from build123d import *

# Parameters (mm, degrees)
F1_DEPTH = 28.575


# Not quite as in the source:
# - a feature names something its author has since deleted; it is built from what else it names


with BuildPart() as f1:
    # F0 (on Top) → F1 (new body)
    with BuildSketch(Plane.XY):
        with BuildLine():
            Line((1102.0184274855, 685.8), (-1143, 685.8))
            Line((-1143, 685.8), (-1143, 0))
            Line((-1143, 0), (88.9, 0))
            Line((88.9, 0), (88.9, 124.587))
            Line((88.9, 124.587), (292.1, 124.587))
            Line((292.1, 124.587), (292.1, 0))
            Line((292.1, 0), (1143, 0))
            Line((1143, 0), (1295.4, 0))
            ThreePointArc((1295.4, 0), (1261.244047213, 330.8283905438), (1160.2171388114, 647.7))
            ThreePointArc((1160.2171388114, 647.7), (1136.7988098871, 675.4279116849), (1102.0184274855, 685.8))
        make_face()
        with BuildLine():
            Line((88.9, 0), (-1143, 0))
            Line((-1143, 0), (-1143, -685.8))
            Line((-1143, -685.8), (1102.0184274855, -685.8))
            ThreePointArc((1102.0184274855, -685.8), (1136.7988098871, -675.4279116849), (1160.2171388114, -647.7))
            ThreePointArc((1160.2171388114, -647.7), (1261.244047213, -330.8283905438), (1295.4, 0))
            Line((1295.4, 0), (1143, 0))
            Line((1143, 0), (292.1, 0))
            Line((292.1, 0), (292.1, -124.587))
            Line((292.1, -124.587), (88.9, -124.587))
            Line((88.9, -124.587), (88.9, 0))
        make_face()
    extrude(amount=F1_DEPTH)


solid = f1.part
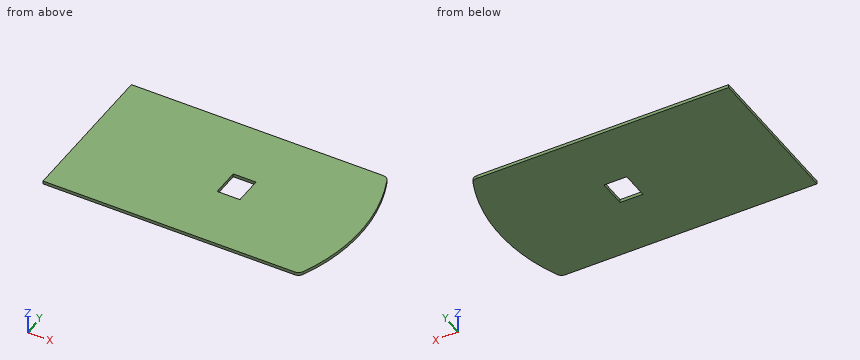
Can you work these out from the model? Positions are in its coordinate system, mm. Give positions to 0.01 mm unless a question says otherwise; leave off trailing zeros. Loops run counter-clockwise (first coordinate to the right, second up) from the corner with the lowest first, then second, coordinate; pieces in that order, holes last. Notation, with made-up numbers: M 70.25,17 L 112.25,17 A36 ccw 112.25,54 Z; hole C -23,10.5 d8. An arc over 180 degrees is marked long. One line per item, written item: value.
1) Imagine slicing it at A-A on z = 10. Write out the boundary of the cut face in (x, y).
Geometry check:
outline: M -1143,-685.8 L 1102.02,-685.8 A63.5 ccw 1160.22,-647.7 A1619.25 ccw 1160.22,647.7 A63.5 ccw 1102.02,685.8 L -1143,685.8 Z; hole M 88.9,-124.59 L 292.1,-124.59 L 292.1,124.59 L 88.9,124.59 Z
2) Imagine slicing it at D-D on y = -502. Write out the boundary of the cut face in (x, z) (3 decimals), and give its area (3 significant figures).
Geometry check:
outline: M -1143,0 L 1215.62,0 L 1215.62,28.575 L -1143,28.575 Z
area: 67,400 mm²
3) Imagine slicing it at C-C on y = 573. Write out the boundary of the cut face in (x, z) (3 decimals).
Geometry check:
outline: M -1143,0 L 1190.627,0 L 1190.627,28.575 L -1143,28.575 Z
4) Imagine slicing it at B-B on y = -96. Write out the boundary of the cut face in (x, z) (3 decimals).
Geometry check:
outline: M -1143,0 L 88.9,0 L 88.9,28.575 L -1143,28.575 Z; M 292.1,0 L 1292.552,0 L 1292.552,28.575 L 292.1,28.575 Z
5) Please list where these lines run through material, in increasing order: line 1 (X direction, y = 109, z = 24); line 2 (Y direction, x = 130, z = 27.75); line 3 (X direction, y = 84.5, z = 22.75).
Geometry check:
line 1: x = -1143 to 88.9, 292.1 to 1291.73
line 2: y = -685.8 to -124.59, 124.59 to 685.8
line 3: x = -1143 to 88.9, 292.1 to 1293.19
